Autodesk Inventor part; units mm, degrees
ref_plane "pins_to_header_XY" through (0, 0, 0) normal (0, 1, 0) x (1, 0, 0)
ref_plane "pins_to_header_YZ" through (0, 0, 0) normal (1, 0, 0) x (0, 0, -1)
ref_plane "pins_to_header_ZX" through (0, 0, 0) normal (0, 0, -1) x (0, 1, 0)
sketch "Sketch_2" plane through (0, 0, 0) normal (1, 0, 0) x (0, 1, 0)
  line L0 (7.5883, 0.0635) -> (-2.8893, 0.0635)
  line L1 (-2.8893, 0.0635) -> (-3.048, -0.0953)
  line L2 (-3.048, -0.0953) -> (-3.048, -0.4128)
  line L3 (-3.048, -0.4128) -> (-2.8893, -0.5715)
  line L4 (-2.8893, -0.5715) -> (7.5883, -0.5715)
  line L5 (7.5883, -0.5715) -> (7.747, -0.4128)
  line L6 (7.747, -0.4128) -> (7.747, -0.0953)
  line L7 (7.747, -0.0953) -> (7.5883, 0.0635)
extrude "Extrusion1" add sketch "Sketch_2" along normal mid plane 3.175
sketch "Sketch_10" plane through (0, 0, 0) normal (0, 0, 1) x (1, 0, 0)
  line L0 (-3.4925, -3.556) -> (4.1275, -3.556)
  line L1 (4.1275, -3.556) -> (4.1275, -3.048)
  line L2 (4.1275, -3.048) -> (3.4925, -3.048)
  line L3 (3.4925, -3.048) -> (3.4925, 1.016)
  line L4 (3.4925, 1.016) -> (1.5875, 1.016)
  line L5 (1.5875, 1.016) -> (1.5875, -3.048)
  line L6 (1.5875, -3.048) -> (0.9525, -3.048)
  line L7 (0.9525, -3.048) -> (0.9525, 1.016)
  line L8 (0.9525, 1.016) -> (-0.9525, 1.016)
  line L9 (-0.9525, 1.016) -> (-0.9525, -3.048)
  line L10 (-0.9525, -3.048) -> (-1.5875, -3.048)
  line L11 (-1.5875, -3.048) -> (-1.5875, 1.016)
  line L12 (-1.5875, 1.016) -> (-3.4925, 1.016)
  line L13 (-3.4925, 1.016) -> (-3.4925, -3.556)
extrude "Extrusion2" cut sketch "Sketch_10" along normal mid plane 6.096
sketch "Sketch_22" plane through (0, 0, 0) normal (0, 0, 1) x (1, 0, 0)
  line L0 (-3.4925, 9.652) -> (-3.4925, 1.524)
  line L1 (-3.4925, 1.524) -> (-1.5875, 1.524)
  line L2 (-1.5875, 1.524) -> (-1.5875, 9.144)
  line L3 (-1.5875, 9.144) -> (-0.9525, 9.144)
  line L4 (-0.9525, 9.144) -> (-0.9525, 1.524)
  line L5 (-0.9525, 1.524) -> (0.9525, 1.524)
  line L6 (0.9525, 1.524) -> (0.9525, 9.144)
  line L7 (0.9525, 9.144) -> (1.5875, 9.144)
  line L8 (1.5875, 9.144) -> (1.5875, 1.524)
  line L9 (1.5875, 1.524) -> (3.4925, 1.524)
  line L10 (3.4925, 1.524) -> (3.4925, 9.144)
  line L11 (3.4925, 9.144) -> (4.1275, 9.144)
  line L12 (4.1275, 9.144) -> (4.1275, 9.652)
  line L13 (4.1275, 9.652) -> (-3.4925, 9.652)
extrude "Extrusion3" cut sketch "Sketch_22" along normal mid plane 6.096
ref_plane "pins_to_header_XY" through (0, 0, 0) normal (0, 1, 0) x (1, 0, 0)
ref_plane "pins_to_header_YZ" through (0, 0, 0) normal (1, 0, 0) x (0, 0, -1)
ref_plane "pins_to_header_ZX" through (0, 0, 0) normal (0, 0, -1) x (0, 1, 0)
properties part number "T-1S64-01-02-S"
Source: CAD feature listing. Evaluate the final solid. Frame: model axes, mm. Coordinates: 2 decimals unless noted, no trailing zeros. Loops run counter-clockwise (first coordinate to the right, second up) from the corner with the lowest first, then second, coordinate; pieces in that order, holes last. Notation, with made-up numbers: (88.25, -12) -> (119.25, -12) arc R20 cw to (119.25, 10) -> close; hole circle Ø7 at (74, -32). An arc over 180 degrees is marked (long way). One line per item, written item: value. Start each with the question number.
Q1. Section query A-A, the plane y = 5.25. Return the cut outline in (x, z).
Q2. Section query C-C, the plane x = 0.75. Return the cut outline in (y, z).
Q3. Line query: line 1 along X through (y, z) = (5.75, -0.15); line 2 along Y through (x, z) = (-0.2, -0.15); line 3 along Y through (x, z) = (-1.3, -0.05). Output: solid intervals per line, ascending.
Q4. Section query B-B, the plane z = -0.3. Return the cut outline in (x, y), and give its area (3 significant figures).
Results:
1. outline: (-1.59, -0.57) -> (-0.95, -0.57) -> (-0.95, 0.06) -> (-1.59, 0.06) -> close; (0.95, -0.57) -> (1.59, -0.57) -> (1.59, 0.06) -> (0.95, 0.06) -> close
2. outline: (1.02, -0.57) -> (1.52, -0.57) -> (1.52, 0.06) -> (1.02, 0.06) -> close
3. line 1: -1.59 to -0.95, 0.95 to 1.59
3. line 2: 1.02 to 1.52
3. line 3: -3 to 7.7
4. outline: (-1.59, -3.05) -> (-0.95, -3.05) -> (-0.95, 1.02) -> (0.95, 1.02) -> (0.95, -3.05) -> (1.59, -3.05) -> (1.59, 7.75) -> (0.95, 7.75) -> (0.95, 1.52) -> (-0.95, 1.52) -> (-0.95, 7.75) -> (-1.59, 7.75) -> close
4. area: 14.7 mm^2
